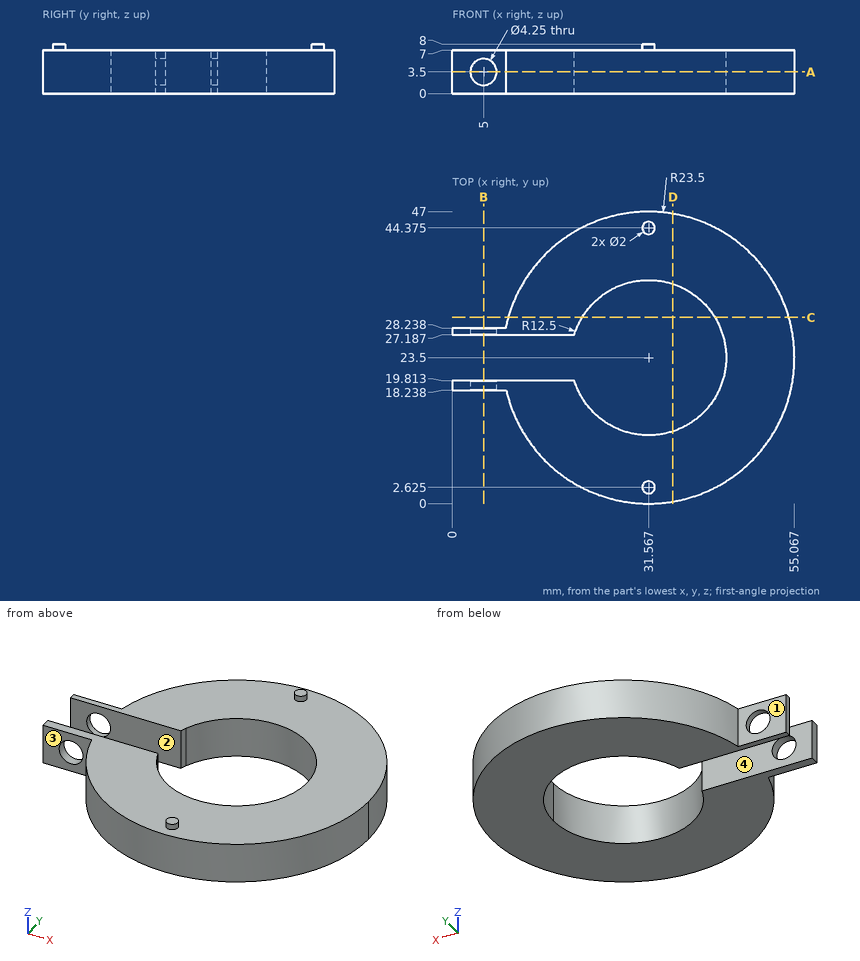
Design review of the part shown in the three views and the two pictorial views. Dimensions are in mm from the part's minimum x, y and z. Coordinates: 2 decimals unless noted, no trailing zeros. Loops run counter-clockwise (first coordinate to the right, second up) from the corner with the lowest first, then second, coordinate; pieces in that order, holes last.
(1) Consider section C-C, the plane y = 30. Give the boundary of the cut face in (x, z), plus the area to 3 significant figures.
Determined:
outline: (8.98, 0) - (20.89, 0) - (20.89, 7) - (8.98, 7) - close; (42.24, 0) - (54.15, 0) - (54.15, 7) - (42.24, 7) - close
area: 167 mm2
(2) Draft analysis for pull direction Y (two halves, no side actions). For the marked faces 1, 2, 3 and 4, state which applies: +Y half, -Y half, draft (parallel to the pull), parting line (faces both ways), or undercut.
Determined:
face 1: +Y half
face 2: undercut
face 3: -Y half
face 4: undercut
(3) Consider section B-B, the plane x = 5. Give the boundary of the cut face in (y, z) (1 decimal).
Determined:
outline: (18.2, 0) - (19.8, 0) - (19.8, 1.4) - (18.2, 1.4) - close; (18.2, 5.6) - (19.8, 5.6) - (19.8, 7) - (18.2, 7) - close; (27.2, 0) - (28.2, 0) - (28.2, 1.4) - (27.2, 1.4) - close; (27.2, 5.6) - (28.2, 5.6) - (28.2, 7) - (27.2, 7) - close
(4) Consider section A-A, the plane z = 3.5. Give the number of separate pieces and of enclosed holes in the cut face, plus the area to 3 significant figures.
Determined:
separate pieces: 3
enclosed holes: 0
area: 1,170 mm2
(5) Wall thickness on L1, parallel to Z at x = 5, y = 18.7 (1 decimal); L2, parallel to Y at x = 37, z = 3.5; L3, parallel to Y at x = 12, z = 6.75 (1 decimal): over which ranges is each line inside the solid? List them lowest first.
Determined:
L1: z = 0 to 1.4, 5.6 to 7
L2: y = 0.64 to 12.24, 34.76 to 46.36
L3: y = 10.5 to 19.8, 27.2 to 36.5
(6) Consider section D-D, the plane x = 35.5. Give the boundary of the cut face in (y, z) (1 decimal), plus the area to 3 significant figures.
Determined:
outline: (0.3, 0) - (11.6, 0) - (11.6, 7) - (0.3, 7) - close; (35.4, 0) - (46.7, 0) - (46.7, 7) - (35.4, 7) - close
area: 158 mm2
(7) Insertion check: P1, Ø3.5, axis at x = 8, z = 2.5, coming from the -Y side (1 decimal); P2, Ø1.5, axis at x = 38, y = 32, coming from the -Z side; P3, Ø1.5, axis at y = 35, z = 2, coming from the -X side; P4, Ø1, axis at y = 29.5, z = 2, coming from the +X side (1 decimal). Each pin has a flat end and moves straight along its axis. Give the tip position at first contact, or say it passes through.
Determined:
P1: stops at y = 14.8
P2: passes through
P3: stops at x = 10.67
P4: stops at x = 54.4
